Autodesk Inventor part; units mm, degrees
ref_plane "YZ Plane" through (0, 0, 0) normal (1, 0, 0) x (0, 1, 0)
ref_plane "XZ Plane" through (0, 0, 0) normal (0, 1, 0) x (-1, 0, 0)
ref_plane "XY Plane" through (0, 0, 0) normal (0, 0, 1) x (1, 0, 0)
sketch "Náčrt1" plane through (0, 0, 0) normal (0, 0, 1) x (1, 0, 0)
  line L0 (0, 7) -> (0, -7)
  line L1 (-7, 0) -> (7, 0)
  line L2 (-3.5, 3.5) -> (3.5, 3.5)
  line L3 (3.5, 3.5) -> (3.5, -3.5)
  line L4 (3.5, -3.5) -> (-3.5, -3.5)
  line L5 (-3.5, -3.5) -> (-3.5, 3.5)
  line L6 (-5, 5) -> (5, 5)
  line L7 (5, 5) -> (5, -5)
  line L8 (5, -5) -> (-5, -5)
  line L9 (-5, -5) -> (-5, 5)
  point P0 (0, 0)
  dimension "d1" = 10
  dimension "d2" = 10
  dimension "d3" = 1.5
  dimension "d4" = 1.5
  dimension "d5" = 1.5
  dimension "d6" = 1.5
extrude "Vysunutí1" add sketch "Náčrt1" along normal mid plane 12.5 contours L6 L7 L1 L3 L2 L0 | L0 L2 L5 L1 L9 L6 | L1 L5 L4 L0 L8 L9 | L7 L8 L0 L4 L3 L1
sketch "Náčrt2" plane through (-5, 5, 6.25) normal (0, 1, 0) x (1, 0, 0)
  line L0 (12, 6.25) -> (-2, 6.25)
  line L1 (5, 15) -> (5, -2.5)
  line L2 (10, 0) -> (0, 0)
  line L3 (0, 12.5) -> (0, 0)
  point P0 (5, 6.25)
  point P1 (5, 5)
  dimension "d10" = 5
  dimension "d11" = 5
hole "Díra1" at (0, 5, 1.25) direction (0, -1, 0) diameter 3.2 end through all
mirror "Zrcadlit1" about plane through (0, 0, -6.25) normal (0, 0, -1) of "Vysunutí1", "Díra1"
properties part number "bearing_standoff" material "Hliník 6061"
Here's how the part is built. I have some questions about the finished solid (model axes, mm). A direction names the side the tool comes from. Coordinates: 2 decimals unless noted, no trailing zeros. Write each loop counter-clockwise with the first axis right and the second up, starting at its lowest first coordinate (ties: lowest second). Pieces come first, ordered by that corner, then holes.
1) If we section it at A-A (x = -2.75): List the corners of the cut face in (y, z) for me.
Filled in:
outline: (-5, -18.75) - (-3.5, -18.75) - (-3.5, 6.25) - (-5, 6.25) - close; (3.5, -18.75) - (5, -18.75) - (5, 6.25) - (3.5, 6.25) - close
2) If I drill on line 1 (Z direction, x = 0, y = 4.4); line 2 (Y direction, x = 0, z = -1.25), over which ranges is the centre line in solid material (lowest first)?
Filled in:
line 1: z = -18.75 to -15.35, -12.15 to -0.35, 2.85 to 6.25
line 2: y = -5 to -3.5, 3.5 to 5
3) If we section it at D-D (x = 0): List the corners of the cut face in (y, z) for me.
Filled in:
outline: (-5, -18.75) - (-3.5, -18.75) - (-3.5, -15.35) - (-5, -15.35) - close; (-5, -12.15) - (-3.5, -12.15) - (-3.5, -0.35) - (-5, -0.35) - close; (-5, 2.85) - (-3.5, 2.85) - (-3.5, 6.25) - (-5, 6.25) - close; (3.5, -18.75) - (5, -18.75) - (5, -15.35) - (3.5, -15.35) - close; (3.5, -12.15) - (5, -12.15) - (5, -0.35) - (3.5, -0.35) - close; (3.5, 2.85) - (5, 2.85) - (5, 6.25) - (3.5, 6.25) - close
4) Thinking about a two-plate mould opening in Y: for faces 1 (the face through (-5, 0, -6)), 2 (the face through (0, 5, -6)), 3 (the face through (-3.5, 0, -6)), which applies, +Y half, -Y half, draft (parallel to the pull), parting line (faces both ways), or undercut?
Filled in:
face 1: draft
face 2: +Y half
face 3: undercut
5) If we section it at B-B (z = -13.75): List the corners of the cut face in (x, y) for me.
Filled in:
outline: (-5, -5) - (-1.6, -5) - (-1.6, -3.5) - (-3.5, -3.5) - (-3.5, 3.5) - (-1.6, 3.5) - (-1.6, 5) - (-5, 5) - close; (1.6, -5) - (5, -5) - (5, 5) - (1.6, 5) - (1.6, 3.5) - (3.5, 3.5) - (3.5, -3.5) - (1.6, -3.5) - close
6) I'm going to push a flat-ended pin straight in: pin 1 (3 mm diameter, centred on x = 0, z = -13.75, fed in from -Y). Where does the tip first touch, or does it pass through?
Filled in:
pin 1: passes through
7) Which directions (+Z, -Z, +X, -X, +Y, -Y) give clear straight access to the entire face, cutting with the end or side of a thin tool? Please do faces 4 (the face through (0, -5, -6)), 5 (the face through (0, -3.5, -6)).
Filled in:
face 4: +Z, -Z, +X, -X, -Y
face 5: +Z, -Z
